Geometry: see drawing. Coordinates: mm, zero at the bounding-box minimum. A direction names the side the tool comes from. Coordinates: 2 decimals unless noted, no trailing zeros. Order: outer loops, then holes, each group sorted by start corner. A loop starts at its lowest first (then second) coordinate and runs counter-clockwise, first axis right, second up.
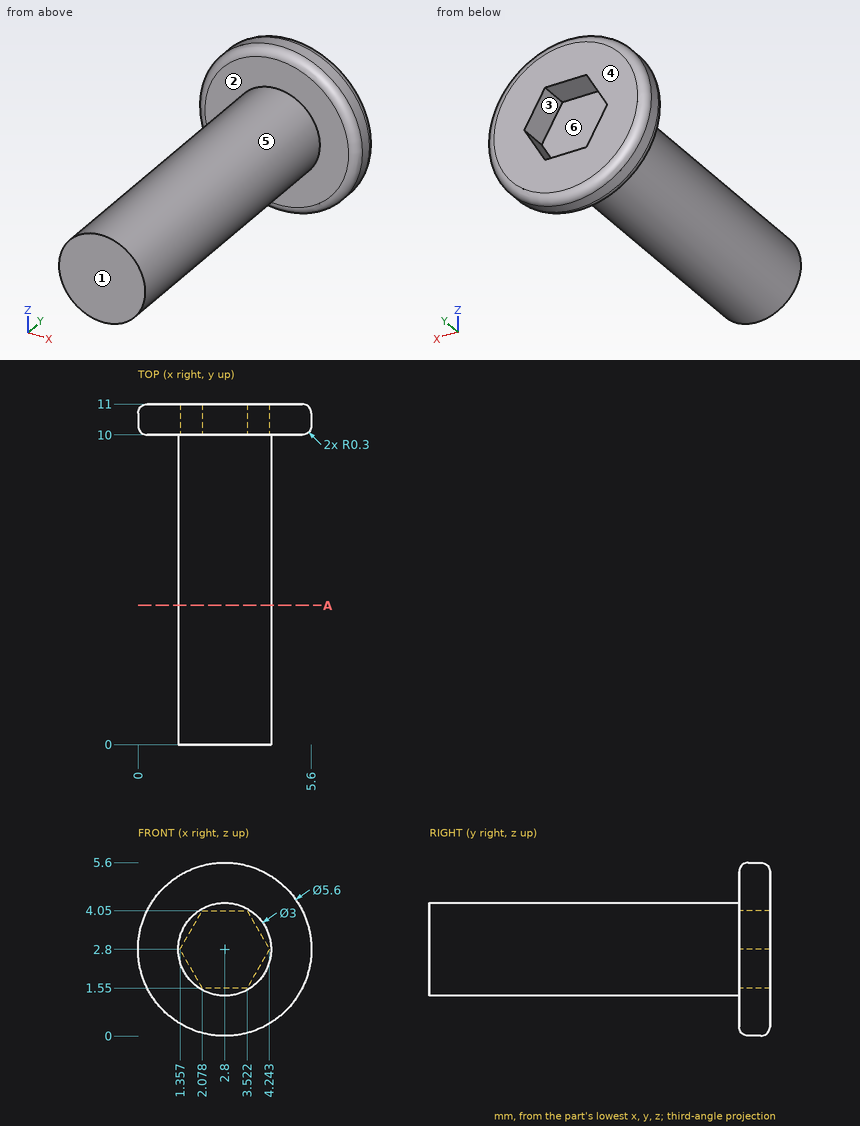
Item 1: Draft query along Z for the marked faces 4, 5 and 6. Return one class per face: pulls with the +Z half, pulls with the -Z half, needs draft (parallel to the pull), parting line crosses it, or undercut.
Response values:
face 4: needs draft
face 5: parting line crosses it
face 6: undercut
Item 2: Ray query, probe 1 along Y at (x, z) = (2.5, 5); probe 2 along Y at (x, z) = (3.4, 3.15); probe 3 along Z at (x, y) = (2.75, 6.5). Return the intervals inside material, ascending.
Response values:
probe 1: y = 10 to 11
probe 2: y = 0 to 10
probe 3: z = 1.3 to 4.3
Item 3: Access query for the marked faces 1, 2 and 3. Directions: +Z, -Z, +X, -X, +Y, -Y. A direction counts if a zero-diameter tool reaches every point of the face in a straight line with its end or side. Return the directions, or none.
Response values:
face 1: +Z, -Z, +X, -X, -Y
face 2: -Y
face 3: +Y
Item 4: Pin query (flat end, axial travel): pin 1 Ø1 at (x, z) = (2.5, 2.5) entering from +Y; pin 2 Ø1.5 at (x, y) = (4, 3) entering from +Z; pin 3 Ø1.5 at (x, y) = (2, 4.5) entering from -Z. Return the tip coordinate at first contact, or that it passes through.
Response values:
pin 1: stops at y = 10
pin 2: stops at z = 4.23
pin 3: stops at z = 1.3
Item 5: Cut plane A-A on y = 4.5. Return loops of the section in (x, z).
Response values:
outline: circle Ø3 at (2.8, 2.8)
